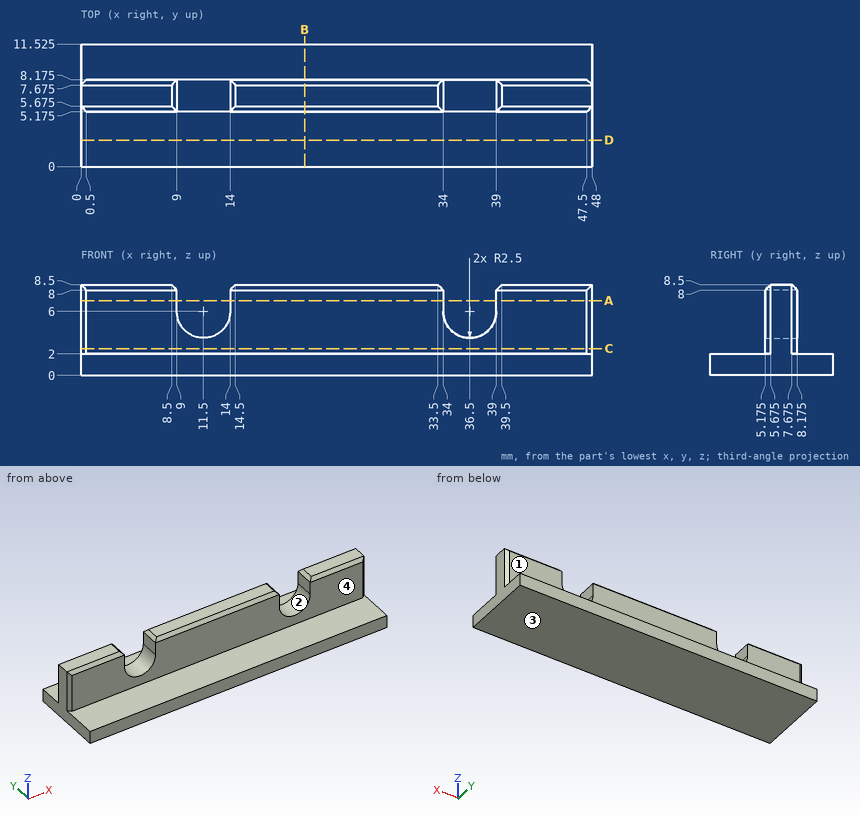
Geometry: see drawing. Coordinates: mm, zero at the bounding-box minimum. A direction names the side the tool comes from. Give positions to 0.01 mm unless a question says otherwise; leave off trailing zeros. Order: outer loops, then holes, each group sorted by start corner. A loop starts at its lowest first (then second) coordinate and runs counter-clockwise, first axis right, second up. Notation, with made-up numbers: (18.25, 89) -> (48.25, 89) arc R15 ccw to (48.25, 105) -> close; hole circle Ø10 at (67, -29.5). An arc over 180 degrees is marked (long way). Write each question's results on one line, items separated by ' | '.
1) Draft query along X for the marked faces 1 and 2. Return one class per face: released by +X, released by -X, zero draft, split by the parting line, or undercut.
Geometry says:
face 1: zero draft | face 2: undercut
2) Cut plane B-B (x = 21). Output: boundary loops of the cut face in (y, z) (3 decimals).
Geometry says:
outline: (0, 0) -> (11.525, 0) -> (11.525, 2) -> (8.175, 2) -> (8.175, 8) -> (7.675, 8.5) -> (5.675, 8.5) -> (5.175, 8) -> (5.175, 2) -> (0, 2) -> close
3) Line query: line 1 along X through (y, z) = (6.5, 7.25); line 2 along X through (y, z) = (5.5, 3.75) (3 decimals); line 3 along Z through (x, y) = (46, 4.75). Output: solid intervals per line, ascending.
Geometry says:
line 1: x = 0 to 9, 14 to 34, 39 to 48 | line 2: x = 0.175 to 10.41, 12.59 to 35.41, 37.59 to 47.825 | line 3: z = 0 to 2
4) Cut plane A-A (z = 7). Output: boundary loops of the cut face in (x, y) (3 decimals).
Geometry says:
outline: (0, 5.675) -> (0.5, 5.175) -> (9, 5.175) -> (9, 8.175) -> (0.5, 8.175) -> (0, 7.675) -> close; (14, 5.175) -> (34, 5.175) -> (34, 8.175) -> (14, 8.175) -> close; (39, 5.175) -> (47.5, 5.175) -> (48, 5.675) -> (48, 7.675) -> (47.5, 8.175) -> (39, 8.175) -> close
5) First-contact query: pin 1 Ø2 at (y, z) = (9, 7) entering from +X (3 decimals); pin 2 Ø3 at (x, z) = (14.5, 5.5) entering from -Y (3 decimals); pin 3 Ø1 at (x, y) = (36, 9.5) entering from +Z. Flat tips, straight axial feed; report the tip coordinate or a pass-through.
Geometry says:
pin 1: stops at x = 47.675 | pin 2: stops at y = 5.175 | pin 3: stops at z = 2
6) Set-up query: the marked faces 3 and 4. Return all of +Z, -Z, +X, -X, +Y, -Y with unobstructed straight access to the full face (end or side cutting, diameter ignored); none if empty.
Geometry says:
face 3: -Z, +X, -X, +Y, -Y | face 4: +Z, +X, -X, -Y
7) Cut plane C-C (z = 2.5). Output: boundary loops of the cut face in (x, y) (3 decimals), and give its area (4 significant figures).
Geometry says:
outline: (0, 5.675) -> (0.5, 5.175) -> (47.5, 5.175) -> (48, 5.675) -> (48, 7.675) -> (47.5, 8.175) -> (0.5, 8.175) -> (0, 7.675) -> close | area: 143.5 mm²
8) Cut plane D-D (y = 2.5). Output: boundary loops of the cut face in (x, z), and give its area (3 significant figures).
Geometry says:
outline: (0, 0) -> (48, 0) -> (48, 2) -> (0, 2) -> close | area: 96.0 mm²
